Design review of the part built by this model. Coordinates are the model's own, in mm. Face numbers are marked on the shaded views. A direction names the side the tool comes from. Coordinates: 2 decimals unless noted, no trailing zeros. Order: outer loops, then holes, each group sorted by start corner. A loop starts at its lowest first (then second) coordinate and runs counter-clockwise, first axis right, second up. Notation, with made-up numbers: (48, -21.75) -> (52, -21.75) arc R23 ccw to (52, 17.25) -> close; hole circle Ø11 at (64.5, 63.25). An arc over 180 degrees is marked (long way). Write item = value, one per line.
```python
from build123d import *

# Parameters (mm, degrees)
F1_DEPTH = 101.6
F4_DEPTH = 25.401
F5_DEPTH = 76.2


with BuildPart() as f1:
    # F0 (on Front) → F1 (new body, symmetric)
    with BuildSketch(Plane.XZ):
        Polygon((0, 25.4), (0, 0), (127, 0), (177.8, 50.8), (228.6, 0), (254, 25.4), (127, 152.4), (101.6, 127), (152.475678, 76.124322), (101.751356, 25.4), align=None)
    extrude(amount=F1_DEPTH, both=True)

    # F3 (on face) → F4 (cut, through all)
    with BuildSketch(Plane.XY.offset(25.4)):
        with BuildLine():
            Line((50.8, 25.4), (0, 25.4))
            Line((0, 25.4), (0, -25.4))
            Line((0, -25.4), (50.8, -25.4))
            ThreePointArc((50.8, -25.4), (76.2, 0), (50.8, 25.4))
        make_face()
    extrude(amount=-F4_DEPTH, mode=Mode.SUBTRACT)

    # F2 (on face) → F5 (cut)
    with BuildSketch(Plane(origin=(139.7, 0, 139.7), x_dir=(0, 1, 0), z_dir=(0.707107, 0, 0.707107))):
        with BuildLine():
            ThreePointArc((50.8, -45.539488), (76.2, -20.139488), (50.8, 5.260512))
            Line((50.8, 5.260512), (-50.8, 5.260512))
            ThreePointArc((-50.8, 5.260512), (-76.2, -20.139488), (-50.8, -45.539488))
            Line((-50.8, -45.539488), (50.8, -45.539488))
        make_face()
        with BuildLine():
            Line((-50.8, -148.94461), (50.8, -148.94461))
            ThreePointArc((50.8, -148.94461), (76.2, -123.54461), (50.8, -98.14461))
            Line((50.8, -98.14461), (-50.8, -98.14461))
            ThreePointArc((-50.8, -98.14461), (-76.2, -123.54461), (-50.8, -148.94461))
        make_face()
    extrude(amount=-F5_DEPTH, mode=Mode.SUBTRACT)


solid = f1.part
```
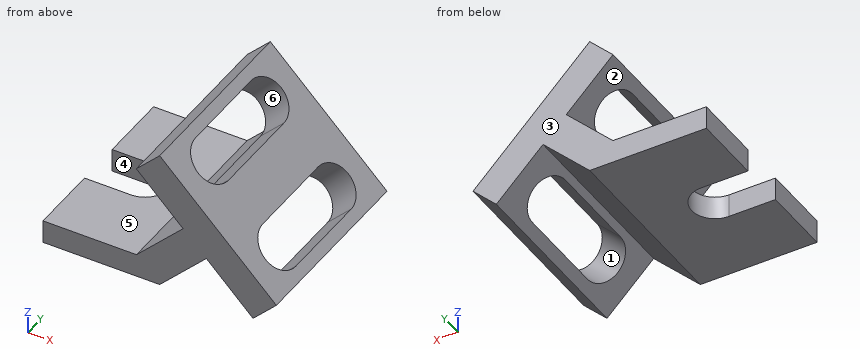
(1) For the marked faces 4, 5 and 6, list the 3-axis set-ups (+Z, -Z, +X, -X, +Y, -Y) from which the entire face can be reached by the end or side of a thin tool; tool diameter is ignored.
Report:
face_4 = +Z, -Z, -X
face_5 = +Z, -X, +Y, -Y
face_6 = none
(2) For L1, parallel to Z at x = 132.5, y = -45; L2, parallel to Y at x = 162.5, z = 116.5; L3, parallel to Z at x = 35, y = 65.5, list the stretches that pass through material, from the lowest coordinate up.
Report:
L1 = 5.5 to 56.15, 139.94 to 146.9
L2 = -101.6 to -72.97, 72.97 to 101.6
L3 = 0 to 25.4
(3) We need section A-A (x = 37.5). Write out the cut boundary in (y, z).
Report:
outline = (-101.6, 0) -> (-25.4, 0) -> (-25.4, 25.4) -> (-101.6, 25.4) -> close; (25.4, 0) -> (101.6, 0) -> (101.6, 25.4) -> (25.4, 25.4) -> close
(4) We need section C-C (y = 84). Write out the cut boundary in (x, z).
Report:
outline = (0, 0) -> (127, 0) -> (177.8, 50.8) -> (228.6, 0) -> (254, 25.4) -> (127, 152.4) -> (101.6, 127) -> (152.48, 76.12) -> (101.75, 25.4) -> (0, 25.4) -> close
(5) The part is to be moulded in two halves that separate along X. For the marked faces 1, 2 and 3, say which applies: released by +X, released by -X, zero draft, split by the parting line, or undercut.
Report:
face_1 = undercut
face_2 = released by -X
face_3 = zero draft
(6) Insertion check: pin 1 (8 mm diameter, centred on y = 59, z = 57, fed in from -X); pin 2 (8 mm diameter, centred on x = 223.5, y = 75.5, fed in from +Z); pin 3 (3 mm diameter, centred on x = 94.5, y = -54, fed in from +Z). Each pin has a flat end and moves straight along its axis. Give the tip position at first contact, or say it passes through.
Report:
pin_1 = 129.35
pin_2 = 59.9
pin_3 = 25.4
(7) We need section B-B (y = 0). Write out the cut boundary in (x, z), and give its area (3 significant figures).
Report:
outline = (76.2, 0) -> (127, 0) -> (177.8, 50.8) -> (183.7, 44.9) -> (209.1, 70.3) -> (171.9, 107.5) -> (146.5, 82.1) -> (152.48, 76.12) -> (101.75, 25.4) -> (76.2, 25.4) -> close; (101.6, 127) -> (110.58, 118.02) -> (135.98, 143.42) -> (127, 152.4) -> close; (219.62, 8.98) -> (228.6, 0) -> (254, 25.4) -> (245.02, 34.38) -> close
area = 6,340 mm²
